The listing builds one solid part. Answer for the finished solid, in the listing's coordinates (mm). A direction names the side the tool comes from. Round coordinates to 2 decimals unless told otherwise and drop trailing zeros. Write each loop counter-clockwise with the first axis right and the second up, starting at its lowest first coordinate (ties: lowest second). Pieces come first, ordered by that corner, then holes.
from build123d import *

# Parameters (mm, degrees)
F0_W           = 31.2
F0_H           = 9
F1_DEPTH       = 25
F3_D           = 17.2
F5_D           = 4
F5_CBORE_D     = 6.7
F5_CBORE_DEPTH = 3
F6_R           = 1


with BuildPart() as f1:
    # F0 (on Right) → F1 (new body)
    with BuildSketch(Plane.YZ):
        Polygon((-7, 0), (0, 0), (0, 60), (-7, 60), (-7, 9), align=None)
        with Locations((-22.6, 4.5)):
            Rectangle(F0_W, F0_H)
    extrude(amount=-F1_DEPTH)

    # F3 (through all)
    with Locations(Plane.XY.offset(9)):
        with Locations((-12.5, -24.6)):
            Hole(F3_D / 2)

    # F5 (through all)
    with Locations(Plane.XZ.offset(7)):
        with Locations((-11.5, 51)):
            CounterBoreHole(F5_D / 2, F5_CBORE_D / 2, F5_CBORE_DEPTH)

    # F6
    f6_edges = [f1.edges().sort_by_distance(p)[0] for p in [
        (-12.5, -7, 9),
    ]]
    fillet(f6_edges, radius=F6_R)


solid = f1.part
1. Section B-B on x = -4.75 is taken. Determine the outline of the cut face in (y, z).
Geometry says:
outline: (-38.2, 0) - (-28.33, 0) - (-28.33, 9) - (-38.2, 9) - close; (-20.87, 0) - (0, 0) - (0, 60) - (-7, 60) - (-7, 10) arc R1 cw to (-8, 9) - (-20.87, 9) - close
2. For a pull along Y with two mould halves and no side action, classify faces 1 (the face through (-12, -7, 35)), 2 (the face through (-11.38, -16.073, 4.437)), 3 (the face through (-25, -6, 21)) as released by +Y, released by -Y, zero draft, split by the parting line, or undercut.
Geometry says:
face 1: released by -Y
face 2: undercut
face 3: zero draft
3. Given pin 1 (3.5 mm diameter, centred on x = -11.5, z = 51, fed in from -Y); pin 2 (6 mm diameter, centred on x = -10.5, z = 44.5, fed in from -Y), each flat-ended and moving along its own axis, determine where each tip first touches the part or whether it passes through.
Geometry says:
pin 1: passes through
pin 2: stops at y = -7
4. Section D-D on x = -11.5 is taken. Determine the outline of the cut face in (y, z), plus the area to 3 significant figures.
Geometry says:
outline: (-38.2, 0) - (-33.14, 0) - (-33.14, 9) - (-38.2, 9) - close; (-16.06, 0) - (0, 0) - (0, 49) - (-4, 49) - (-4, 47.65) - (-7, 47.65) - (-7, 10) arc R1 cw to (-8, 9) - (-16.06, 9) - close; (-7, 54.35) - (-4, 54.35) - (-4, 53) - (0, 53) - (0, 60) - (-7, 60) - close
area: 511 mm2
5. Section A-A on z = 51 is taken. Determine the outline of the cut face in (x, y).
Geometry says:
outline: (-25, -7) - (-14.85, -7) - (-14.85, -4) - (-13.5, -4) - (-13.5, 0) - (-25, 0) - close; (-9.5, -4) - (-8.15, -4) - (-8.15, -7) - (0, -7) - (0, 0) - (-9.5, 0) - close
6. Section C-C on y = -28 is taken. Determine the outline of the cut face in (x, z), plus the area to 3 significant figures.
Geometry says:
outline: (-25, 0) - (-20.4, 0) - (-20.4, 9) - (-25, 9) - close; (-4.6, 0) - (0, 0) - (0, 9) - (-4.6, 9) - close
area: 82.8 mm2
7. Straight lines are drawn through the part: line 1 along Y through (x, z) = (-12.5, 7.25); line 2 along Y through (x, z) = (-16.25, 43); line 3 along Z through (x, y) = (-0.75, -20). For each, find the intervals that lie inside material, in ascending order.
Geometry says:
line 1: y = -38.2 to -33.2, -16 to 0
line 2: y = -7 to 0
line 3: z = 0 to 9
8. A tool of negligible diameter and unlimited length cuts with its end or side. For faces 4 (the face through (-12, 0, 30)), 5 (the face through (-7, -17, 9)), 6 (the face through (-9, -4, 51)), from which of +Z, -Z, +X, -X, +Y, -Y can it reach the whole face along a straight path? Write none if from no direction.
Geometry says:
face 4: +Z, -Z, +X, -X, +Y
face 5: +Z, +X, -X, -Y
face 6: -Y
